from build123d import *
from build123d.topology import SkipClean

# Parameters (mm, degrees)
BOSS_EXTRUDE1_DEPTH      = 3
BOSS_EXTRUDE1_DEPTH_BACK = 1.5
SKETCH1_R                = 8
SKETCH2_W                = 16
SKETCH2_H                = 50
BOSS_EXTRUDE2_DEPTH      = 1.5
CUT_EXTRUDE1_REACH       = 52.836
SKETCH3_R                = 1.25
CUT_EXTRUDE3_REACH       = 52.725
SKETCH5_R                = 1.5


with BuildPart() as part:
    # Sketch1 → Boss-Extrude1 (new, two sides: drawn at the far end of the back side and taken through both)
    with BuildSketch(Plane(origin=(0, 0, 0), x_dir=(1, 0, 0), z_dir=(0, 1, 0)).offset(-BOSS_EXTRUDE1_DEPTH_BACK)):
        with Locations(Location((0, 0, 0), (0, 0, 270))):
            Circle(SKETCH1_R)
    extrude(amount=BOSS_EXTRUDE1_DEPTH + BOSS_EXTRUDE1_DEPTH_BACK)

    # Sketch2 → Boss-Extrude2 (add, symmetric)
    with BuildSketch(Plane(origin=(0, 0, 0), x_dir=(1, 0, 0), z_dir=(0, 1, 0))):
        with Locations((0, -25)):
            Rectangle(SKETCH2_W, SKETCH2_H)
    extrude(amount=BOSS_EXTRUDE2_DEPTH, both=True)

    # Sketch3 → Cut-Extrude1 (cut, up to next)
    with BuildSketch(Plane(origin=(0, -1.5, 0), x_dir=(-1, 0, 0), z_dir=(0, -1, 0)), mode=Mode.PRIVATE) as cut_extrude1_sk1:
        with Locations(Location((2.503073418, -45.5, 0), (0, 0, 90))):
            Circle(SKETCH3_R)
    cut_extrude1_tool1 = extrude(cut_extrude1_sk1.sketch, amount=-CUT_EXTRUDE1_REACH, mode=Mode.PRIVATE) & part.part
    # Sketch3 → Cut-Extrude1 (cut, up to next)
    with BuildSketch(Plane(origin=(0, -1.5, 0), x_dir=(-1, 0, 0), z_dir=(0, -1, 0)), mode=Mode.PRIVATE) as cut_extrude1_sk2:
        with Locations(Location((-2.503073418, -45.5, 0), (0, 0, 90))):
            Circle(SKETCH3_R)
    cut_extrude1_tool2 = extrude(cut_extrude1_sk2.sketch, amount=-CUT_EXTRUDE1_REACH, mode=Mode.PRIVATE) & part.part
    add(cut_extrude1_tool1.solids().sort_by_distance((-2.503073, -1.5, 45.5))[0], mode=Mode.SUBTRACT)
    add(cut_extrude1_tool2.solids().sort_by_distance((2.503073, -1.5, 45.5))[0], mode=Mode.SUBTRACT)

    # Sketch4 → Cut-Revolve21 (revolve, cut)
    with SkipClean():  # the faces are left unmerged after this step: merging them gives an invalid solid
        with BuildSketch(Plane(origin=(0, -1.5, 0), x_dir=(-1, 0, 0), z_dir=(0, -1, 0))):
            with BuildLine():
                ThreePointArc((3.3, 0), (0, 3.3), (-3.3, 0))
                Line((-3.3, 0), (3.3, 0))
            make_face()
            with BuildLine():
                Line((3.3, 0), (-3.3, 0))
                ThreePointArc((-3.3, 0), (0, -3.3), (3.3, 0))
            make_face()
        revolve(axis=Axis((3.3, -1.5, 0), (-1, 0, 0)), mode=Mode.SUBTRACT)
    add(part.part.scale(1), mode=Mode.REPLACE)  # the faces are merged on a copy

    # Sketch5 → Cut-Extrude3 (cut, up to next)
    with BuildSketch(Plane(origin=(0, 1.5, 0), x_dir=(1, 0, 0), z_dir=(0, 1, 0)), mode=Mode.PRIVATE) as cut_extrude3_sk1:
        with Locations(Location((0, -25, 0), (0, 0, 270))):
            Circle(SKETCH5_R)
    cut_extrude3_tool1 = extrude(cut_extrude3_sk1.sketch, amount=-CUT_EXTRUDE3_REACH, mode=Mode.PRIVATE) & part.part
    add(cut_extrude3_tool1.solids().sort_by_distance((0, 1.5, 25))[0], mode=Mode.SUBTRACT)


solid = part.part
Build history of the part. All positions in model axes, mm. A direction names the side the tool comes from. Round coordinates to 2 decimals unless told otherwise and drop trailing zeros. Write each loop counter-clockwise with the first axis right and the second up, starting at its lowest first coordinate (ties: lowest second). Pieces come first, ordered by that corner, then holes. Notation, with made-up numbers: M -37.5,41 L 8.5,41 A10 ccw 8.5,48 Z; hole C 74.5,21 d11. An arc over 180 degrees is marked long. Answer in a Markdown table with one row per item.
1. Saw through at C-C (x = -5.75). List the corners of the cut face in (y, z), and give its area (3 significant figures).
Geometry check:
| item | result |
|---|---|
| outline | M -1.5,-5.56 L 3,-5.56 L 3,5.56 L 1.5,5.56 L 1.5,50 L -1.5,50 Z |
| area | 183 mm2 |
2. Saw through at B-B (y = 0.85). List the corners of the cut face in (x, z).
Geometry check:
| item | result |
|---|---|
| outline | M -8,0 A8 ccw 8,0 L 8,50 L -8,50 Z; hole C -2.5,45.5 d2.5; hole C 0,0 d4.63; hole C 0,25 d3; hole C 2.5,45.5 d2.5 |
3. Probe L1, parallel to X at y = 0.65, z = 45.5; L2, parallel to X at y = 0.35, z = 25; L3, parallel to Z at x = -1, y = 0.35. List the from-to ranges inside material, lowest first. Write a range as [from, to].
Geometry check:
| item | result |
|---|---|
| L1 | [-8, -3.75], [-1.25, 1.25], [3.75, 8] |
| L2 | [-8, -1.5], [1.5, 8] |
| L3 | [-7.94, -2.54], [2.54, 23.88], [26.12, 50] |
4. Saw through at A-A (z = 25). List the corners of the cut face in (x, y).
Geometry check:
| item | result |
|---|---|
| outline | M -8,-1.5 L -1.5,-1.5 L -1.5,1.5 L -8,1.5 Z; M 1.5,-1.5 L 8,-1.5 L 8,1.5 L 1.5,1.5 Z |
5. Flat gauge pins, fed straight in: P1, Ø3, axis at x = -2.5, z = 45.5, coming from the -Y side; P2, Ø3, axis at x = -5, z = 18, coming from the +Y side. Where does each tip first touch, or does it go through?
Geometry check:
| item | result |
|---|---|
| P1 | y = -1.5 |
| P2 | y = 1.5 |
6. Mould opens along X. For faces 3 (the face through (-3.264, -0.021, 46.492)), 4 (the face through (-8, 0, 25)), 5 (the face through (0, 3, 0)) say: +X half, -X half, draft (parallel to the pull), parting line (faces both ways), or undercut.
Geometry check:
| item | result |
|---|---|
| face 3 | undercut |
| face 4 | -X half |
| face 5 | draft |
7. Which spindle directions (+Z, -Z, +X, -X, +Y, -Y) get a long thin tool onto all of the face, cutting with end or side? Do faces 1 (the face through (0, 1, -8)), 2 (the face through (8, 0, 25)). Say none if no direction does.
Geometry check:
| item | result |
|---|---|
| face 1 | +Y |
| face 2 | +Z, -Z, +X, +Y, -Y |
8. Saw through at D-D (z = -1.5). List the corners of the cut face in (x, y).
Geometry check:
| item | result |
|---|---|
| outline | M -7.86,-1.5 L -2.94,-1.5 A2.94 cw 2.94,-1.5 L 7.86,-1.5 L 7.86,3 L -7.86,3 Z |
